from build123d import *

# Parameters (mm, degrees)
F0_W     = 40
F0_H     = 10
F1_DEPTH = 12.5
F2_DEPTH = 5
F3_R     = 5


with BuildPart() as f1:
    # F0 (on Front) → F1 (new body, symmetric)
    with BuildSketch(Plane.XZ):
        Polygon((0, 50), (0, 0), (10, 0), (10, 10), (10, 50), align=None)
        with Locations((30, 5)):
            Rectangle(F0_W, F0_H)
    extrude(amount=F1_DEPTH, both=True)

    # F0 (on Front) → F2 (join, symmetric)
    with BuildSketch(Plane.XZ):
        Polygon((10, 50), (10, 10), (50, 10), align=None)
    extrude(amount=F2_DEPTH, both=True)

    # F3
    f3_edges = [f1.edges().sort_by_distance(p)[0] for p in [
        (50, -12.5, 5),
        (50, 12.5, 5),
        (5, 12.5, 50),
        (5, -12.5, 50),
    ]]
    fillet(f3_edges, radius=F3_R)


solid = f1.part
Can you work these out from the model? Positions are in its coordinate system, mm. A direction names the side the tool comes from. Coordinates: 2 decimals unless noted, no trailing zeros. Order: outer loops, then holes, each group sorted by start corner. A loop starts at its lowest first (then second) coordinate and runs counter-clockwise, first axis right, second up. Notation, with made-up numbers: (-7.5, -34.75) - (22.5, -34.75) arc R27 cw to (22.5, -2.75) - close; hole circle Ø3 at (-18.75, 56). An arc over 180 degrees is marked (long way). Answer as a JSON object with one key per item and string values. Group by question number.
Q1. On a 3-axis mill with a long thin cutter (end or side, diameter ignored), from which of +Z, -Z, +X, -X, +Y, -Y can I reach the whole of each face in a straight line? I mean faces 1 (the face through (30, -9, 10)), 2 (the face through (10, 9, 30)), 3 (the face through (30, 0, 30)). Say none if no direction works.
Q2. I need wall thicknesses on line 1 (Z direction, x = 32.5, y = -7); line 2 (Y direction, x = 30.5, z = 29). Which ranges of each line are inside material? Lowest first, please. Write a range as from..to.
Q3. Will these pins go through, and if not, where does the flat tip stop? P1, Ø2, axis at x = 14.5, y = 2, coming from the +Z side; P2, Ø5, axis at x = 15, z = 13, coming from the +Y side; P3, Ø2, axis at x = 12, y = -7.5, coming from the +Z side.
Q4. Imagine slicing it at C-C (y = -6.5). Please give me the cut outline in (x, z).
Q5. Imagine slicing it at B-B (z = 35). Please give me the cut outline in (x, y).
Q6. Imagine slicing it at A-A (x = 37). Please give me the cut outline in (y, z), and give its area (3 significant figures).
Q7. Imagine slicing it at D-D (y = -3.75). Please give me the cut outline in (x, z), and give its area (3 significant figures).
Determined:
{
 "1": {"face 1": "+Z, +X, -Y", "face 2": "+Z, +X, +Y", "face 3": "+Z, +X, +Y, -Y"},
 "2": {"line 1": "z = 0..10", "line 2": "y = -5..5"},
 "3": {"P1": "stops at z = 46.5", "P2": "stops at y = 5", "P3": "stops at z = 10"},
 "4": {"outline": "(0, 0) - (50, 0) - (50, 10) - (10, 10) - (10, 50) - (0, 50) - close"},
 "5": {"outline": "(0, -12.5) - (10, -12.5) - (10, -5) - (25, -5) - (25, 5) - (10, 5) - (10, 12.5) - (0, 12.5) - close"},
 "6": {"outline": "(-12.5, 0) - (12.5, 0) - (12.5, 10) - (5, 10) - (5, 23) - (-5, 23) - (-5, 10) - (-12.5, 10) - close", "area": "380 mm2"},
 "7": {"outline": "(0, 0) - (50, 0) - (50, 10) - (10, 50) - (0, 50) - close", "area": "1,700 mm2"}
}
